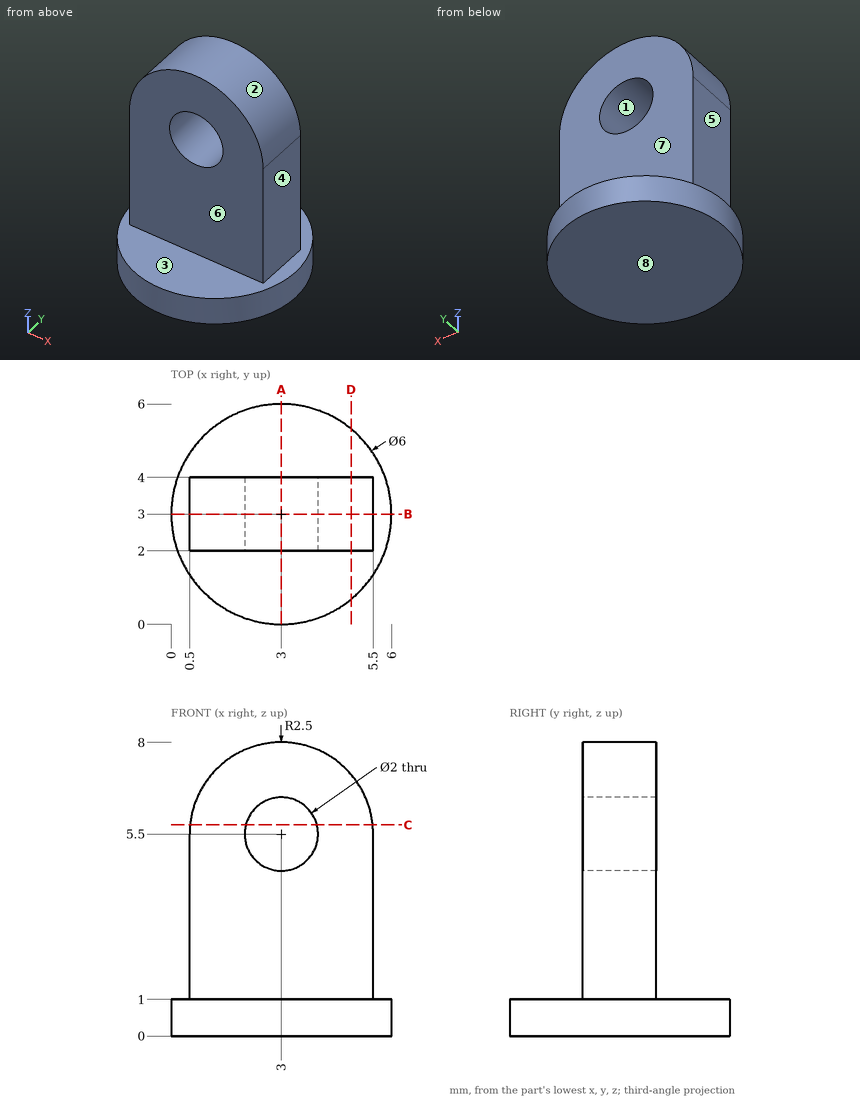
Geometry: see drawing. Coordinates: mm, zero at the bounding-box minimum. A direction names the side the tool comes from. Round coordinates to 2 decimals unless told otherwise and drop trailing zeros. Loops run counter-clockwise (first coordinate to the right, second up) from the corner with the lowest first, then second, coordinate; pieces in that order, holes last. Notation, with made-up numbers: M 60,-5 L 81,-5 A16 ccw 81,-1 Z; hole C 55.25,-25.75 d10. An arc over 180 degrees is marked long. Use a Markdown table: item, result. Add a question column.
1. Mould query, pull axis X, two halves, no side actions, for the marked faces 1, 2, 3 and 4. Classes: pulls with the +X half, pulls with the -X half, needs draft (parallel to the pull), parting line crosses it, or undercut.
2. Section query D-D on x = 4.9. Return the cut outline in (y, z).
3. Section query C-C on z = 5.75. Return the cut outline in (x, y), then the cut area to 3 significant figures.
4. Contact query for flat-ended pins moving along their axis: P1, Ø1, axis at x = 4, z = 3.5, coming from the -Y side; P2, Ø2, axis at y = 3.5, z = 3.5, coming from the +X side; P3, Ø1.6, axis at y = 2.5, z = 4, coming from the -X side. Output: stop coordinate, or through.
5. Section query B-B on y = 3. Return the cut outline in (x, z), then the cut area to 3 significant figures.
6. Line query: line 1 (Z direction, x = 3, y = 2.8); line 2 (Y direction, x = 1.25, z = 4.5); line 3 (X direction, y = 3.95, z = 1.5). Output: solid intervals per line, ascending.
7. Reachability of the marked faces 5, 6, 7 and 8 from +Z, -Z, +X, -X, +Y, -Y: full face, straight path, thin tool, end or side. Return the list, or none.
8. Section query A-A on x = 3. Return the cut outline in (y, z).
Reported:
| question | item | result |
|---|---|---|
| 1 | face 1 | undercut |
| 1 | face 2 | parting line crosses it |
| 1 | face 3 | needs draft |
| 1 | face 4 | pulls with the +X half |
| 2 | outline | M 0.68,0 L 5.32,0 L 5.32,1 L 4,1 L 4,7.12 L 2,7.12 L 2,1 L 0.68,1 Z |
| 3 | outline | M 0.51,2 L 2.03,2 L 2.03,4 L 0.51,4 Z; M 3.97,2 L 5.49,2 L 5.49,4 L 3.97,4 Z |
| 3 | area | 6.08 mm² |
| 4 | P1 | stops at y = 2 |
| 4 | P2 | stops at x = 5.5 |
| 4 | P3 | stops at x = 0.5 |
| 5 | outline | M 0,0 L 6,0 L 6,1 L 5.5,1 L 5.5,5.5 A2.5 ccw 0.5,5.5 L 0.5,1 L 0,1 Z; hole C 3,5.5 d2 |
| 5 | area | 35.2 mm² |
| 6 | line 1 | z = 0 to 4.5, 6.5 to 8 |
| 6 | line 2 | y = 2 to 4 |
| 6 | line 3 | x = 0.5 to 5.5 |
| 7 | face 5 | +Z, -X, +Y, -Y |
| 7 | face 6 | +Z, +X, -X, -Y |
| 7 | face 7 | +Z, +X, -X, +Y |
| 7 | face 8 | -Z, +X, -X, +Y, -Y |
| 8 | outline | M 0,0 L 6,0 L 6,1 L 4,1 L 4,4.5 L 2,4.5 L 2,1 L 0,1 Z; M 2,6.5 L 4,6.5 L 4,8 L 2,8 Z |
